Check sheet for the modelled part. Datum: model origin and axes. Units: mm. Round coordinates to 2 decimals unless told otherwise and drop trailing zeros. Write item = value, one per line.
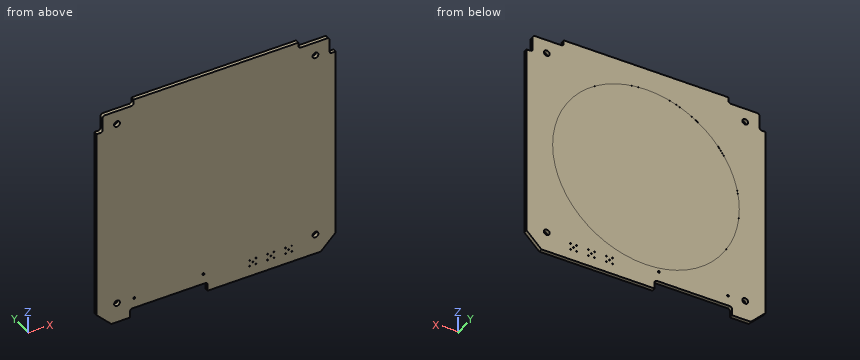
from build123d import *

# Parameters (mm, degrees)
SKETCH1_R                = 0.4
SKETCH1_R_2              = 0.2125
BOSS_EXTRUDE1_DEPTH      = 1.56
SKETCH2_R                = 38.5
CUT_EXTRUDE1_DEPTH       = 0.01
M2_CLEARANCE_HOLE2_D     = 2.4
M2_CLEARANCE_HOLE2_DEPTH = 38.1
M2_CLEARANCE_HOLE2_TIP   = 0.721032743


with BuildPart() as part:
    # Sketch1 → Boss-Extrude1 (new body)
    with BuildSketch(Plane(origin=(0, 0, 0), x_dir=(1, 0, 0), z_dir=(0, 1, 0))):
        with BuildLine():
            Line((-49.356685196, 41.604788024), (-43.256685196, 47.704788024))
            Line((-43.256685196, 47.704788024), (-35.556685196, 47.704788024))
            Line((-35.556685196, 47.704788024), (-35.556685196, 45.004788024))
            ThreePointArc((-35.556685196, 45.004788024), (-35.263791977, 44.297681243), (-34.556685196, 44.004788024))
            Line((-34.556685196, 44.004788024), (-4.556685196, 44.004788024))
            ThreePointArc((-4.556685196, 44.004788024), (-3.849578415, 44.297681243), (-3.556685196, 45.004788024))
            Line((-3.556685196, 45.004788024), (-3.556685196, 47.704788024))
            Line((-3.556685196, 47.704788024), (43.143314804, 47.704788024))
            Line((43.143314804, 47.704788024), (49.243314804, 41.604788024))
            Line((49.243314804, 41.604788024), (49.243314804, -37.995211976))
            Line((49.243314804, -37.995211976), (47.743314804, -37.995211976))
            ThreePointArc((47.743314804, -37.995211976), (47.036208023, -38.288105194), (46.743314804, -38.995211976))
            Line((46.743314804, -38.995211976), (46.743314804, -44.095211976))
            ThreePointArc((46.743314804, -44.095211976), (46.450421585, -44.802318757), (45.743314804, -45.095211976))
            Line((45.743314804, -45.095211976), (34.943314804, -45.095211976))
            ThreePointArc((34.943314804, -45.095211976), (34.236208023, -45.388105194), (33.943314804, -46.095211976))
            Line((33.943314804, -46.095211976), (33.943314804, -47.595211976))
            Line((33.943314804, -47.595211976), (-34.056685196, -47.595211976))
            Line((-34.056685196, -47.595211976), (-34.056685196, -46.095211976))
            ThreePointArc((-34.056685196, -46.095211976), (-34.349578415, -45.388105194), (-35.056685196, -45.095211976))
            Line((-35.056685196, -45.095211976), (-45.856685196, -45.095211976))
            ThreePointArc((-45.856685196, -45.095211976), (-46.563791977, -44.802318757), (-46.856685196, -44.095211976))
            Line((-46.856685196, -44.095211976), (-46.856685196, -38.995211976))
            ThreePointArc((-46.856685196, -38.995211976), (-47.149578415, -38.288105194), (-47.856685196, -37.995211976))
            Line((-47.856685196, -37.995211976), (-49.356685196, -37.995211976))
            Line((-49.356685196, -37.995211976), (-49.356685196, 41.604788024))
        make_face()
        with Locations(Location((-33.826685196, 39.744788024, 0), (0, 0, 270))):
            Circle(SKETCH1_R, mode=Mode.SUBTRACT)
        with Locations(Location((-5.276685196, 39.744788024, 0), (0, 0, 270))):
            Circle(SKETCH1_R, mode=Mode.SUBTRACT)
        with Locations(Location((29.883314804, 42.004788024, 0), (0, 0, 270))):
            Circle(SKETCH1_R_2, mode=Mode.SUBTRACT)
        with Locations(Location((28.613314804, 43.274788024, 0), (0, 0, 270))):
            Circle(SKETCH1_R_2, mode=Mode.SUBTRACT)
        with Locations(Location((31.153314804, 43.274788024, 0), (0, 0, 270))):
            Circle(SKETCH1_R_2, mode=Mode.SUBTRACT)
        with Locations(Location((31.153314804, 40.734788024, 0), (0, 0, 270))):
            Circle(SKETCH1_R_2, mode=Mode.SUBTRACT)
        with Locations(Location((28.613314804, 40.734788024, 0), (0, 0, 270))):
            Circle(SKETCH1_R_2, mode=Mode.SUBTRACT)
        with Locations(Location((22.483314804, 42.004788024, 0), (0, 0, 270))):
            Circle(SKETCH1_R_2, mode=Mode.SUBTRACT)
        with Locations(Location((21.213314804, 43.274788024, 0), (0, 0, 270))):
            Circle(SKETCH1_R_2, mode=Mode.SUBTRACT)
        with Locations(Location((23.753314804, 43.274788024, 0), (0, 0, 270))):
            Circle(SKETCH1_R_2, mode=Mode.SUBTRACT)
        with Locations(Location((23.753314804, 40.734788024, 0), (0, 0, 270))):
            Circle(SKETCH1_R_2, mode=Mode.SUBTRACT)
        with Locations(Location((21.213314804, 40.734788024, 0), (0, 0, 270))):
            Circle(SKETCH1_R_2, mode=Mode.SUBTRACT)
        with Locations(Location((15.083314804, 42.004788024, 0), (0, 0, 270))):
            Circle(SKETCH1_R_2, mode=Mode.SUBTRACT)
        with Locations(Location((13.813314804, 43.274788024, 0), (0, 0, 270))):
            Circle(SKETCH1_R_2, mode=Mode.SUBTRACT)
        with Locations(Location((16.353314804, 43.274788024, 0), (0, 0, 270))):
            Circle(SKETCH1_R_2, mode=Mode.SUBTRACT)
        with Locations(Location((16.353314804, 40.734788024, 0), (0, 0, 270))):
            Circle(SKETCH1_R_2, mode=Mode.SUBTRACT)
        with Locations(Location((13.813314804, 40.734788024, 0), (0, 0, 270))):
            Circle(SKETCH1_R_2, mode=Mode.SUBTRACT)
    extrude(amount=BOSS_EXTRUDE1_DEPTH)

    # Sketch2 → Cut-Extrude1 (cut)
    with BuildSketch(Plane(origin=(0, 1.56, 0), x_dir=(1, 0, 0), z_dir=(0, 1, 0))):
        with Locations(Location((0, 0, 0), (0, 0, 270))):
            Circle(SKETCH2_R)
    extrude(amount=-CUT_EXTRUDE1_DEPTH, mode=Mode.SUBTRACT)

    # M2 Clearance Hole2
    with Locations(Plane(origin=(0, 1.56, 0), x_dir=(1, 0, 0), z_dir=(0, 1, 0))):
        with Locations((-40.929491149, 39.39737116), (40.929491149, 39.39737116), (40.929491149, -39.39737116), (-40.929491149, -39.39737116)):
            Hole(M2_CLEARANCE_HOLE2_D / 2, depth=M2_CLEARANCE_HOLE2_DEPTH)
            with Locations((0, 0, -(M2_CLEARANCE_HOLE2_DEPTH + M2_CLEARANCE_HOLE2_TIP / 2))):  # 118° drill point
                Cone(0, M2_CLEARANCE_HOLE2_D / 2, M2_CLEARANCE_HOLE2_TIP, mode=Mode.SUBTRACT)


solid = part.part
(1) Material ranges on L1, parallel to Z at x = -40.5, y = 0.8; L2, parallel to Y at x = 34.5, z = -4.5; L3, parallel to Z at x = 39, y = 0.95, recorded low to high. Write a range as [from, to].
Worked answers:
L1 = [-47.7, -40.52], [-38.28, 38.28], [40.52, 45.1]
L2 = [0, 1.55]
L3 = [-47.7, 45.1]
(2) Go/stop test with flat-tipped pins: P1, Ø1, axis at x = 29.5, z = 32, coming from the -Y side; P2, Ø23, axis at x = -18, z = 11, coming from the +Y side; P3, Ø0.8, axis at x = 39.5, y = 0.5, coming from the +Z side; P4, Ø0.5, axis at y = 1, z = -46.5, coming from the +X side. Record where each tip stops, or that it passes through.
Worked answers:
P1 = 0
P2 = 1.55
P3 = 45.1
P4 = 44.6
(3) Sectioned sample at B-B on y = 1.15. Count the separate pieces of the cut face and the enclosed holes in it, then the cut area to 3 significant figures.
Worked answers:
separate_pieces = 1
enclosed_holes = 21
area = 9,110 mm²
